CAD build for the part. Positions are in the model's coordinates, mm. Face numbers are marked on the shaded views. A direction names the side the tool comes from. Coordinates: 2 decimals unless noted, no trailing zeros. Loops run counter-clockwise (first coordinate to the right, second up) from the corner with the lowest first, then second, coordinate; pieces in that order, holes last. Notation, with made-up numbers: (45, 22) -> (50, 22) arc R14 cw to (50, 45) -> close; hole circle Ø5 at (-23, -23.75). An arc over 180 degrees is marked (long way). Return JSON: item names as keys, results as strings. Group by question number.
(1) Saw through at B-B on x = 38.1. Write the cut outline in (y, z).
(2) Saw through at C-C on y = -8. Write the cut outline in (x, z).
(3) Saw through at A-A on z = 33.5. Write the cut outline in (x, y).
(4) Flat gauge pins, fed straight in: pin 1 Ø9.5 at (x, y) = (9, -15.5) entering from +Z; pin 2 Ø10 at (x, z) = (-38.1, 44.45) entering from +Y; pin 3 Ø1.5 at (x, z) = (35, 49.5) entering from -Y; pin 4 Ø3.5 at (y, z) = (-24.5, 8) entering from +X. Where does each tip first touch, or does it go through?
(5) Probe L1, parallel to Z at x = -38, y = -9; L2, parallel to X at y = -13, z = 28.5; L3, parallel to Y at x = 2, z = 13.5. List the from-to ranges inside material, lowest first.
(6) Saw through at D-D on z = 41. Write the cut outline in (x, y).
(7) Tool access for the marked faces 4, 5, 6 and 7: list every direction of +Z, -Z, +X, -X, +Y, -Y with a clear straight run to the whole face (end or side of a thin tool).
(8) Mould opens along Z. For the marked faces 1, 2 and 3 say: pulls with the +Z half, pulls with the -Z half, needs draft (parallel to the pull), parting line crosses it, or undercut.
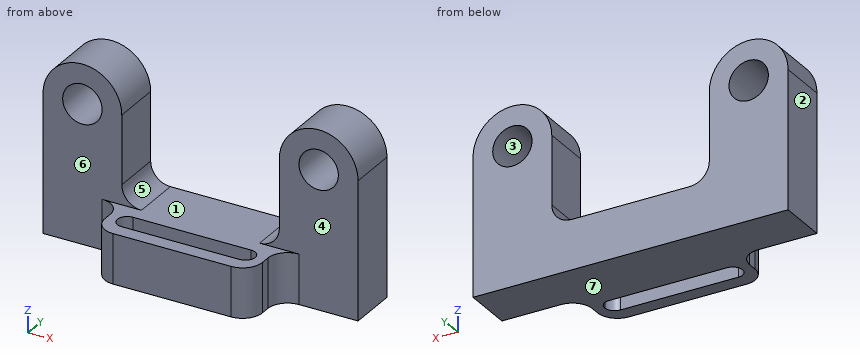
```python
from build123d import *

# Parameters (mm, degrees)
F1_DEPTH = 31.75
F2_W     = 15.748
F2_H     = 28.448
F2_H_2   = 12.7
F3_DEPTH = 101.601
F5_DEPTH = 16.003
F6_R     = 6.35
F7_DEPTH = 16.003
F8_R     = 6.35
F9_DEPTH = 16.003


with BuildPart() as f1:
    # F0 (on Front) → F1 (new body)
    with BuildSketch(Plane.XZ):
        with BuildLine():
            Line((-50.8, 0), (0, 0))
            Line((0, 0), (0, 16.002))
            Line((0, 16.002), (-19.05, 16.002))
            ThreePointArc((-19.05, 16.002), (-23.540128, 17.861872), (-25.4, 22.352))
            Line((-25.4, 22.352), (-25.4, 44.45))
            ThreePointArc((-25.4, 44.45), (-38.1, 57.15), (-50.8, 44.45))
            Line((-50.8, 44.45), (-50.8, 0))
        make_face()
        with BuildLine():
            Line((0, 16.002), (0, 0))
            Line((0, 0), (50.8, 0))
            Line((50.8, 0), (50.8, 44.45))
            ThreePointArc((50.8, 44.45), (38.1, 57.15), (25.4, 44.45))
            Line((25.4, 44.45), (25.4, 22.352))
            ThreePointArc((25.4, 22.352), (23.540128, 17.861872), (19.05, 16.002))
            Line((19.05, 16.002), (0, 16.002))
        make_face()
    extrude(amount=F1_DEPTH)

    # F2 (on face) → F3 (cut, through all)
    with BuildSketch(Plane.YZ.offset(50.8)):
        with Locations((-23.876, 30.226)):
            Rectangle(F2_W, F2_H)
        with Locations((-23.876, 50.8)):
            Rectangle(F2_W, F2_H_2)
    extrude(amount=-F3_DEPTH, mode=Mode.SUBTRACT)

    # F4 (on face) → F5 (cut, through all)
    with BuildSketch(Plane.XY.offset(16.002)):
        with BuildLine():
            Line((-31.75, -16.002), (-50.8, -16.002))
            Line((-50.8, -16.002), (-50.8, -31.75))
            Line((-50.8, -31.75), (-19.05, -31.75))
            ThreePointArc((-19.05, -31.75), (-23.540128, -29.890128), (-25.4, -25.4))
            Line((-25.4, -25.4), (-25.4, -22.352))
            ThreePointArc((-25.4, -22.352), (-27.259872, -17.861872), (-31.75, -16.002))
        make_face()
        with BuildLine():
            ThreePointArc((-19.05, -20.701), (-16.804936, -21.630936), (-15.875, -23.876))
            ThreePointArc((-15.875, -23.876), (-16.804936, -26.121064), (-19.05, -27.051))
            Line((-19.05, -27.051), (19.05, -27.051))
            ThreePointArc((19.05, -27.051), (15.875, -23.876), (19.05, -20.701))
            Line((19.05, -20.701), (-19.05, -20.701))
        make_face()
        with BuildLine():
            ThreePointArc((-19.05, -27.051), (-16.804936, -26.121064), (-15.875, -23.876))
            ThreePointArc((-15.875, -23.876), (-16.804936, -21.630936), (-19.05, -20.701))
            ThreePointArc((-19.05, -20.701), (-22.225, -23.876), (-19.05, -27.051))
        make_face()
        with BuildLine():
            ThreePointArc((22.225, -23.876), (21.295064, -21.630936), (19.05, -20.701))
            Line((19.05, -20.701), (19.05, -27.051))
            ThreePointArc((19.05, -27.051), (21.295064, -26.121064), (22.225, -23.876))
        make_face()
        with BuildLine():
            Line((19.05, -27.051), (19.05, -20.701))
            ThreePointArc((19.05, -20.701), (15.875, -23.876), (19.05, -27.051))
        make_face()
        with BuildLine():
            ThreePointArc((25.4, -25.4), (23.540128, -29.890128), (19.05, -31.75))
            Line((19.05, -31.75), (50.8, -31.75))
            Line((50.8, -31.75), (50.8, -16.002))
            Line((50.8, -16.002), (31.75, -16.002))
            ThreePointArc((31.75, -16.002), (27.259872, -17.861872), (25.4, -22.352))
            Line((25.4, -22.352), (25.4, -25.4))
        make_face()
    extrude(amount=-F5_DEPTH, mode=Mode.SUBTRACT)

    # F6 (on face) → F7 (cut, through all)
    with BuildSketch(Plane.XZ.offset(16.002)):
        with Locations((-38.1, 44.45)):
            Circle(F6_R)
    extrude(amount=-F7_DEPTH, mode=Mode.SUBTRACT)

    # F8 (on face) → F9 (cut, through all)
    with BuildSketch(Plane.XZ.offset(16.002)):
        with Locations((38.1, 44.45)):
            Circle(F8_R)
    extrude(amount=-F9_DEPTH, mode=Mode.SUBTRACT)


solid = f1.part
```
Geometry results:
{
 "1": {"outline": "(-16, 0) -> (0, 0) -> (0, 38.1) -> (-16, 38.1) -> close; (-16, 50.8) -> (0, 50.8) -> (0, 57.15) -> (-16, 57.15) -> close"},
 "2": {"outline": "(-50.8, 0) -> (50.8, 0) -> (50.8, 44.45) arc R12.7 ccw to (25.4, 44.45) -> (25.4, 22.35) arc R6.35 cw to (19.05, 16) -> (-19.05, 16) arc R6.35 cw to (-25.4, 22.35) -> (-25.4, 44.45) arc R12.7 ccw to (-50.8, 44.45) -> close; hole circle Ø12.7 at (-38.1, 44.45); hole circle Ø12.7 at (38.1, 44.45)"},
 "3": {"outline": "(-50.8, -16) -> (-25.4, -16) -> (-25.4, 0) -> (-50.8, 0) -> close; (25.4, -16) -> (50.8, -16) -> (50.8, 0) -> (25.4, 0) -> close"},
 "4": {"pin 1": "z = 16", "pin 2": "through", "pin 3": "y = -16", "pin 4": "x = 25.4"},
 "5": {"L1": "0 to 38.1, 50.8 to 57.15", "L2": "-50.8 to -25.4, 25.4 to 50.8", "L3": "-31.75 to -27.05, -20.7 to 0"},
 "6": {"outline": "(-50.8, -16) -> (-43.43, -16) -> (-43.43, 0) -> (-50.8, 0) -> close; (-32.77, -16) -> (-25.4, -16) -> (-25.4, 0) -> (-32.77, 0) -> close; (25.4, -16) -> (32.77, -16) -> (32.77, 0) -> (25.4, 0) -> close; (43.43, -16) -> (50.8, -16) -> (50.8, 0) -> (43.43, 0) -> close"},
 "7": {"face 4": "+Z, +X, -Y", "face 5": "+Z, +Y, -Y", "face 6": "+Z, -X, -Y", "face 7": "-Z, +X, -X, +Y, -Y"},
 "8": {"face 1": "pulls with the +Z half", "face 2": "needs draft", "face 3": "undercut"}
}
